Check sheet for the modelled part. Datum: model origin and axes. Units: mm. Give positions to 0.01 mm unless a question says otherwise; leave off trailing zeros. Order: outer loops, then holes, each group sorted by start corner. A loop starts at its lowest first (then second) coordinate and runs counter-clockwise, first axis right, second up.
from build123d import *

# Parameters (mm, degrees)
SKETCH2_W                      = 520
SKETCH2_H                      = 450
BOSS_EXTRUDE2_DEPTH            = 10
SKETCH3_W                      = 10.2
SKETCH3_H                      = 100.2
CUT_EXTRUDE1_DEPTH             = 2
FILLET2_R                      = 2
CBORE_FOR_M5_SHCS1_D           = 5.5
CBORE_FOR_M5_SHCS1_CBORE_D     = 10
CBORE_FOR_M5_SHCS1_CBORE_DEPTH = 5
FILLET2_OF_MIRROR8_R           = 2
SKETCH7_W                      = 400
SKETCH7_H                      = 230
CUT_EXTRUDE3_DEPTH             = 11
FILLET3_R                      = 2
SKETCH9_W                      = 420
SKETCH9_H                      = 250
CUT_EXTRUDE5_DEPTH             = 5
FILLET4_R                      = 2
M3_TAPPED_HOLE1_D              = 2.5
CUT_EXTRUDE8_DEPTH             = 6
SKETCH11_W                     = 5
SKETCH11_H                     = 17
CUT_EXTRUDE7_DEPTH             = 261
CUT_EXTRUDE7_DEPTH_BACK        = 261
FILLET1_R                      = 1
M5X0_8_TAPPED_HOLE1_D          = 4.2
M5X0_8_TAPPED_HOLE1_DEPTH      = 8
M5X0_8_TAPPED_HOLE1_TIP        = 1.2618073
SKETCH17_W                     = 19
SKETCH17_H                     = 27
CUT_EXTRUDE9_DEPTH             = 2
FILLET5_R                      = 2
M4X0_7_TAPPED_HOLE1_AT_2_COUNT = 2
M4X0_7_TAPPED_HOLE1_AT_2_PITCH = 15
FILLET5_OF_MIRROR10_R          = 2
F_1_0MM_DOWEL_HOLE1_D          = 1
F_1_0MM_DOWEL_HOLE1_DEPTH      = 4
F_1_0MM_DOWEL_HOLE1_TIP        = 0.30043031


with BuildPart() as part:
    # Sketch2 → Boss-Extrude2 (new body)
    with BuildSketch(Plane.XY):
        with Locations((0, -165)):
            Rectangle(SKETCH2_W, SKETCH2_H)
    extrude(amount=-BOSS_EXTRUDE2_DEPTH)

    # Sketch3 → Cut-Extrude1 (cut)
    with BuildSketch(Plane.XY):
        with Locations((-155.1, 0)):
            Rectangle(SKETCH3_W, SKETCH3_H)
    cut_extrude1 = extrude(amount=-CUT_EXTRUDE1_DEPTH, mode=Mode.SUBTRACT)

    # Fillet2
    fillet2_edges = [part.edges().sort_by_distance(p)[0] for p in [
        (-150, 50.1, -1),
        (-150, -50.1, -1),
        (-160.2, -50.1, -1),
        (-160.2, 50.1, -1),
    ]]
    fillet(fillet2_edges, radius=FILLET2_R)

    # CBORE for M5 SHCS1 (through all)
    with Locations(Plane(origin=(0, 0, -10), x_dir=(-1, 0, 0), z_dir=(0, 0, -1))):
        with Locations((155.1, 25), (155.1, -25)):
            cbore_for_m5_shcs1 = CounterBoreHole(CBORE_FOR_M5_SHCS1_D / 2, CBORE_FOR_M5_SHCS1_CBORE_D / 2, CBORE_FOR_M5_SHCS1_CBORE_DEPTH)

    # Mirror8: Cut-Extrude1, CBORE for M5 SHCS1 across plane
    add(cut_extrude1.mirror(Plane(origin=(0, 0, 0), x_dir=(0, 0, 1), z_dir=(1, 0, 0))), mode=Mode.SUBTRACT)
    add(cbore_for_m5_shcs1.mirror(Plane(origin=(0, 0, 0), x_dir=(0, 0, 1), z_dir=(1, 0, 0))), mode=Mode.SUBTRACT)

    # Fillet2 of Mirror8
    fillet2_of_mirror8_edges = [part.edges().sort_by_distance(p)[0] for p in [
        (150, 50.1, -1),
        (150, -50.1, -1),
        (160.2, -50.1, -1),
        (160.2, 50.1, -1),
    ]]
    fillet(fillet2_of_mirror8_edges, radius=FILLET2_OF_MIRROR8_R)

    # Sketch7 → Cut-Extrude3 (cut, through all)
    with BuildSketch(Plane.XY):
        with Locations((0, -215)):
            Rectangle(SKETCH7_W, SKETCH7_H)
    extrude(amount=-CUT_EXTRUDE3_DEPTH, mode=Mode.SUBTRACT)

    # Fillet3
    fillet3_edges = [part.edges().sort_by_distance(p)[0] for p in [
        (200, -100, -5),
        (200, -330, -5),
        (-200, -330, -5),
        (-200, -100, -5),
    ]]
    fillet(fillet3_edges, radius=FILLET3_R)

    # Sketch9 → Cut-Extrude5 (cut)
    with BuildSketch(Plane.XY):
        with Locations((0, -215)):
            Rectangle(SKETCH9_W, SKETCH9_H)
    extrude(amount=-CUT_EXTRUDE5_DEPTH, mode=Mode.SUBTRACT)

    # Fillet4
    fillet4_edges = [part.edges().sort_by_distance(p)[0] for p in [
        (210, -90, -2.5),
        (210, -340, -2.5),
        (-210, -340, -2.5),
        (-210, -90, -2.5),
    ]]
    fillet(fillet4_edges, radius=FILLET4_R)

    # M3 Tapped Hole1 (through all)
    with Locations(Plane.XY.offset(-5)):
        with Locations((-205, -95), (0, -95), (-205, -215), (205, -95), (205, -215), (205, -335), (0, -335), (-205, -335)):
            Hole(M3_TAPPED_HOLE1_D / 2)

    # Sketch12 → Cut-Extrude8 (cut)
    with BuildSketch(Plane(origin=(0, 0, -10), x_dir=(-1, 0, 0), z_dir=(0, 0, -1))):
        with BuildLine():
            Line((10, -390), (-10, -390))
            Line((-10, -390), (-10, -386.5))
            ThreePointArc((-10, -386.5), (-9.267766953, -384.732233047), (-7.5, -384))
            Line((-7.5, -384), (7.5, -384))
            ThreePointArc((7.5, -384), (9.267766953, -384.732233047), (10, -386.5))
            Line((10, -386.5), (10, -390))
        make_face()
    extrude(amount=-CUT_EXTRUDE8_DEPTH, mode=Mode.SUBTRACT)

    # Sketch11 → Cut-Extrude7 (cut, two sides)
    with BuildSketch(Plane(origin=(0, 0, 0), x_dir=(0, 0, -1), z_dir=(1, 0, 0))) as cut_extrude7_sk:
        Polygon((10, -390), (0, -388.685250563), (0, -390), align=None)
        with Locations((7.5, 51.5)):
            Rectangle(SKETCH11_W, SKETCH11_H)
    extrude(amount=CUT_EXTRUDE7_DEPTH, mode=Mode.SUBTRACT)
    extrude(cut_extrude7_sk.sketch, amount=-CUT_EXTRUDE7_DEPTH_BACK, mode=Mode.SUBTRACT)

    # Fillet1
    fillet1_edges = [part.edges().sort_by_distance(p)[0] for p in [
        (260, 60, -2.5),
        (-260, 60, -2.5),
        (260, -164.342625282, 0),
        (-260, -389.342625282, -5),
        (0, -388.685250563, 0),
        (260, -389.342625282, -5),
        (-260, -164.342625282, 0),
        (0, 60, 0),
    ]]
    fillet(fillet1_edges, radius=FILLET1_R)

    # M5x0.8 Tapped Hole1
    with Locations(Plane(origin=(0, 0, -10), x_dir=(-1, 0, 0), z_dir=(0, 0, -1))):
        with Locations((-215, 34), (-190, 34), (-12.5, 34), (12.5, 34), (190, 34), (215, 34)):
            Hole(M5X0_8_TAPPED_HOLE1_D / 2, depth=M5X0_8_TAPPED_HOLE1_DEPTH)
            with Locations((0, 0, -(M5X0_8_TAPPED_HOLE1_DEPTH + M5X0_8_TAPPED_HOLE1_TIP / 2))):  # 118° drill point
                Cone(0, M5X0_8_TAPPED_HOLE1_D / 2, M5X0_8_TAPPED_HOLE1_TIP, mode=Mode.SUBTRACT)

    # Sketch17 → Cut-Extrude9 (cut)
    with BuildSketch(Plane(origin=(0, 0, -10), x_dir=(-1, 0, 0), z_dir=(0, 0, -1))):
        with Locations((143.85, -376.5)):
            Rectangle(SKETCH17_W, SKETCH17_H)
    cut_extrude9 = extrude(amount=-CUT_EXTRUDE9_DEPTH, mode=Mode.SUBTRACT)

    # Fillet5
    fillet5_edges = [part.edges().sort_by_distance(p)[0] for p in [
        (-153.35, -363, -9),
        (-134.35, -363, -9),
    ]]
    fillet(fillet5_edges, radius=FILLET5_R)

    # Sketch19 → M4x0.7 Tapped Hole1 (revolve, cut)
    with BuildSketch(Plane(origin=(-143.85, -385, -8), x_dir=(0, 1, 0), z_dir=(1, 0, 0))):
        Polygon((0, 0), (0, 6.991420021), (1.65, 6), (1.65, 0), align=None)
    m4x0_7_tapped_hole1 = revolve(axis=Axis((-143.85, -385, -14.35), (0, 0, 1)), mode=Mode.SUBTRACT)

    # M4x0.7 Tapped Hole1 at 2: M4x0.7 Tapped Hole1 ×2
    with Locations(*[(0, i * M4X0_7_TAPPED_HOLE1_AT_2_PITCH, 0) for i in range(1, M4X0_7_TAPPED_HOLE1_AT_2_COUNT)]):
        add(m4x0_7_tapped_hole1, mode=Mode.SUBTRACT)

    # Mirror10: M4x0.7 Tapped Hole1, Cut-Extrude9 across plane
    add(m4x0_7_tapped_hole1.mirror(Plane(origin=(0, 0, 0), x_dir=(0, 0, 1), z_dir=(1, 0, 0))), mode=Mode.SUBTRACT)
    add(cut_extrude9.mirror(Plane(origin=(0, 0, 0), x_dir=(0, 0, 1), z_dir=(1, 0, 0))), mode=Mode.SUBTRACT)

    # Mirror10 copy 1 sketch → Mirror10 copy 1 (revolve, cut)
    with BuildSketch(Plane(origin=(143.85, -370, -8), x_dir=(0, 1, 0), z_dir=(-1, 0, 0))):
        Polygon((0, 0), (0, -6.991420021), (1.65, -6), (1.65, 0), align=None)
    revolve(axis=Axis((143.85, -370, -14.35), (0, 0, -1)), mode=Mode.SUBTRACT)

    # Fillet5 of Mirror10
    fillet5_of_mirror10_edges = [part.edges().sort_by_distance(p)[0] for p in [
        (153.35, -363, -9),
        (134.35, -363, -9),
    ]]
    fillet(fillet5_of_mirror10_edges, radius=FILLET5_OF_MIRROR10_R)

    # Ø1.0mm Dowel Hole1
    with Locations(Plane.XY.offset(-5)):
        with Locations((-205, -155), (205, -275)):
            Hole(F_1_0MM_DOWEL_HOLE1_D / 2, depth=F_1_0MM_DOWEL_HOLE1_DEPTH)
            with Locations((0, 0, -(F_1_0MM_DOWEL_HOLE1_DEPTH + F_1_0MM_DOWEL_HOLE1_TIP / 2))):  # 118° drill point
                Cone(0, F_1_0MM_DOWEL_HOLE1_D / 2, F_1_0MM_DOWEL_HOLE1_TIP, mode=Mode.SUBTRACT)


solid = part.part
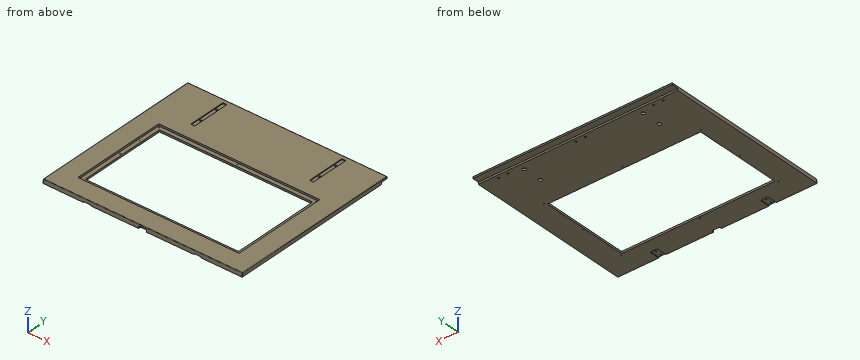
1) Section check B-B, the plane x = 98. Record the cut outline in (y, z).
Recorded:
outline: (-390, -10) - (-330, -10) - (-330, -5) - (-340, -5) - (-340, 0) - (-387.81, 0) arc R1 ccw to (-388.8, -0.87) - close; (-100, -10) - (43, -10) - (43, -5) - (60, -5) - (60, -1) arc R1 ccw to (59, 0) - (-90, 0) - (-90, -5) - (-100, -5) - close
2) Section check A-A, the plane y = -310. Record the cut outline in (x, z), then the cut area to 3 significant figures.
Recorded:
outline: (-260, -10) - (-200, -10) - (-200, -5) - (-210, -5) - (-210, 0) - (-259, 0) arc R1 ccw to (-260, -1) - close; (200, -10) - (260, -10) - (260, -1) arc R1 ccw to (259, 0) - (210, 0) - (210, -5) - (200, -5) - close
area: 1,100 mm2
3) Material ranges on L1, parallel to X at y = -335, z = -7.45; L2, parallel to Y at x = -143.85, z = -4.3; L3, parallel to X at y = -215, z = -7.8, recorded low to high.
Recorded:
L1: x = -260 to -206.25, -203.75 to -1.25, 1.25 to 203.75, 206.25 to 260
L2: y = -389.25 to -386.65, -383.35 to -371.65, -368.35 to -340, -90 to 60
L3: x = -260 to -206.25, -203.75 to -200, 200 to 203.75, 206.25 to 260
4) Depth check by flat-ended pin: pin 1 Ø5 at (x, y) = (-16.5, 53.5) entering from -Z; pin 2 Ø1.5 at (x, z) = (83.5, -2.5) entering from -Y; pin 3 Ø2.5 at (x, z) = (-4, -7.5) entering from +Y. Enter the tip coordinate at first touch or a pass-through.
Recorded:
pin 1: stops at z = -5
pin 2: stops at y = -389.11
pin 3: stops at y = 43
